Check sheet for the drawn part. Datum: minimum x, y, z corner. Units: mm. A direction names the side the tool comes from. Round coordinates to 2 decimals unless told otherwise and drop trailing zeros. Loops run counter-clockwise (first coordinate to the right, second up) from the corner with the lowest first, then second, coordinate; pieces in that order, holes last.
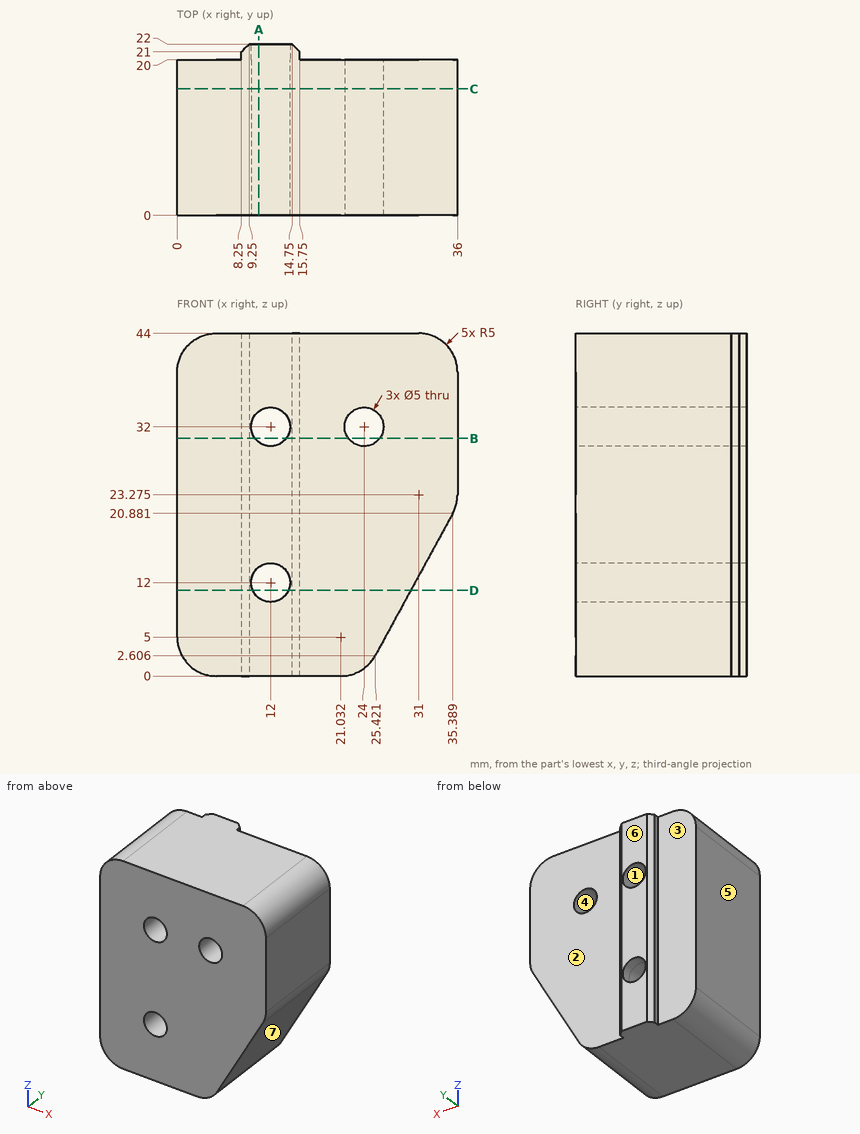
1. Scan lines: L1, parallel to X at y = 15.75, z = 32; L2, parallel to Z at x = 12, y = 14; L3, parallel to X at y = 20.85, z = 12. Record each from-to range of solid material in increasing order.
2. Section check A-A (x = 10.5). Enter the section's corners in (y, z), then the cut area to 3 significant figures.
3. Section check B-B (z = 30.5). Enter the section's corners in (x, y).
4. Tool access check on the marked faces 1, 2 and 3. Record the directions out of +Z, -Z, +X, -X, +Y, -Y that give a thin tool (end or side, any length) a straight path to the whole face; none if there is none.
5. Section check C-C (y = 16.25). Enter the section's corners in (x, z) (1 decimal).
6. Release check for a two-part mould opening along X. For the marked faces 4, 5, 6 and 7 record: released by +X, released by -X, zero draft, split by the parting line, or undercut.
7. Gauge pin test, flat ends, axial feed: P1, Ø2, axis at y = 14, z = 27.5, coming from the -X side; P2, Ø9, axis at x = 4, z = 21, coming from the +Y side; P3, Ø8, axis at x = 31, y = 13.5, coming from the -Z side; P4, Ø3, axis at y = 4.5, z = 11, coming from the +X side. Record the tip position at first contact, or that the pin passes through.
8. Section check D-D (z = 11). Enter the section's corners in (x, y).
Taken from the geometry:
1. L1: x = 0 to 9.5, 14.5 to 21.5, 26.5 to 36
1. L2: z = 0 to 9.5, 14.5 to 29.5, 34.5 to 44
1. L3: x = 8.25 to 9.5, 14.5 to 15.75
2. outline: (0, 0) - (22, 0) - (22, 10) - (0, 10) - close; (0, 14) - (22, 14) - (22, 30) - (0, 30) - close; (0, 34) - (22, 34) - (22, 44) - (0, 44) - close
2. area: 792 mm2
3. outline: (0, 0) - (10, 0) - (10, 22) - (9.25, 22) - (8.25, 21) - (8.25, 20) - (0, 20) - close; (14, 0) - (22, 0) - (22, 20) - (15.75, 20) - (15.75, 21) - (14.75, 22) - (14, 22) - close; (26, 0) - (36, 0) - (36, 20) - (26, 20) - close
4. face 1: +Y, -Y
4. face 2: +Z, -Z, +X, +Y
4. face 3: +Z, -Z, -X, +Y
5. outline: (0, 5) arc R5 ccw to (5, 0) - (21, 0) arc R5 ccw to (25.4, 2.6) - (35.4, 20.9) arc R5 ccw to (36, 23.3) - (36, 39) arc R5 ccw to (31, 44) - (5, 44) arc R5 ccw to (0, 39) - close; hole circle Ø5 at (12, 12); hole circle Ø5 at (12, 32); hole circle Ø5 at (24, 32)
6. face 4: undercut
6. face 5: released by -X
6. face 6: zero draft
6. face 7: released by +X
7. P1: stops at x = 0
7. P2: stops at y = 21.25
7. P3: stops at z = 5.5
7. P4: stops at x = 30.82
8. outline: (0, 0) - (9.71, 0) - (9.71, 22) - (9.25, 22) - (8.25, 21) - (8.25, 20) - (0, 20) - close; (14.29, 0) - (30, 0) - (30, 20) - (15.75, 20) - (15.75, 21) - (14.75, 22) - (14.29, 22) - close
